```python
from build123d import *

# Parameters (mm, degrees)
EXTRUDE1_OUTLINE_R = 4.309736146
EXTRUDE1_DEPTH     = 3
EXTRUDE2_START     = -57
SKETCH2_R          = 4.309736146
EXTRUDE2_DEPTH     = 57


# Read off the part's stored shape, not the designer's step: Extrude1
with BuildPart() as part:
    # Extrude1 outline → Extrude1 (new body)
    with BuildSketch(Plane.XY):
        with BuildLine():
            ThreePointArc((-11.990836263, 60.528054794), (-22.672294112, 59.063871996), (-21.516296681, 48.344681589))
            Line((-21.516296681, 48.344681589), (67.256693566, -25.277180433))
            ThreePointArc((67.256693566, -25.277180433), (83.02731963, -23.576417361), (80.873138344, -7.861305383))
            Line((80.873138344, -7.861305383), (-11.990836263, 60.528054794))
        make_face()
        with Locations((74.315769624, -16.765370586)):
            Circle(EXTRUDE1_OUTLINE_R, mode=Mode.SUBTRACT)
        with Locations((-16.578080379, 54.299165973)):
            Circle(EXTRUDE1_OUTLINE_R, mode=Mode.SUBTRACT)
    extrude(amount=EXTRUDE1_DEPTH)

    # Sketch2 → Extrude2 (add)
    with BuildSketch(Plane.XY.offset(3).offset(EXTRUDE2_START)):
        with Locations((74.315769624, -16.765370586)):
            Circle(SKETCH2_R)
    extrude(amount=EXTRUDE2_DEPTH)


solid = part.part
```
Check sheet for the modelled part. Datum: model origin and axes. Units: mm. A direction names the side the tool comes from. Coordinates: 2 decimals unless noted, no trailing zeros. Order: outer loops, then holes, each group sorted by start corner. A loop starts at its lowest first (then second) coordinate and runs counter-clockwise, first axis right, second up. Notation, with made-up numbers: M 10,26 L 45,26 A6 cw 45,31 Z; hole C 36,62.25 d1. An arc over 180 degrees is marked long. Write each question's results on one line, items separated by ' | '. Start each with the question number.
1. Mould release check, pull along X, two halves, no side actions. Record for faces 1 (the face through (-17.139, 58.572, 1.479)), 2 (the face through (82.87, -23.77, 1.48)), 3 (the face through (34, 17, 0)): +X half, -X half, draft (parallel to the pull), parting line (faces both ways), or undercut.
2. Cross-section at D-D on z = -43.5. Record the cut outline in (x, y), and give its area (3 significant figures).
3. Cross-section at C-C on y = -15.5. Record the cut outline in (x, z).
4. Access from +Z, -Z, +X, -X, +Y, -Y to the whole of each face (thin tool, end or side, straight path). Record for faces 4 (the face through (70.01, -16.58, -27.38)), 5 (the face through (34, 14, 3)).
5. Material ranges on probe 1 along Z at (x, y) = (44, -1); probe 2 along X at (y, z) = (-19, -28.5), recorded low to high.
6. Cross-section at B-B on x = 72. Record the cut outline in (y, z).
7. Go/stop test with a flat-tipped pin: P1, Ø5, axis at x = -16.58, y = 54.3, coming from the +Z side. Record where the tip stops, or that it passes through.
8. Cross-section at A-A on x = -14.5. Record the cut outline in (y, z), and give its area (3 significant figures).
Checks:
1) face 1: undercut | face 2: parting line | face 3: draft
2) outline: C 74.32,-16.77 d8.62 | area: 58.4 mm²
3) outline: M 55.47,0 L 70.2,0 L 70.2,-54 L 78.44,-54 L 78.44,0 L 85.3,0 L 85.3,3 L 55.47,3 Z
4) face 4: -Z | face 5: +Z, +X, -X, +Y, -Y
5) probe 1: z = 0 to 3 | probe 2: x = 70.63 to 78
6) outline: M -27.58,0 L -20.4,0 L -20.4,-54 L -13.13,-54 L -13.13,0 L -1.33,0 L -1.33,3 L -27.58,3 Z
7) P1: passes through
8) outline: M 42.53,0 L 50.52,0 L 50.52,3 L 42.53,3 Z; M 58.07,0 L 61.75,0 L 61.75,3 L 58.07,3 Z | area: 35.0 mm²
